Read the model definition and answer for the solid it produces. Units are mm, in the model's axes. A direction names the side the tool comes from. Coordinates: 2 decimals unless noted, no trailing zeros. Write each loop counter-clockwise with the first axis right and the second up, starting at its lowest first coordinate (ties: lowest second). Pieces come first, ordered by that corner, then holes. Notation, with made-up numbers: (72.25, -7.5) -> (115.25, -7.5) arc R24 cw to (115.25, 26.5) -> close; hole circle Ø6 at (30.25, -13). An arc over 180 degrees is marked (long way). Write item = value, one per line. Start each with the question number.
1) Section A-A (y = 11.43) is taken. Count the separate pieces of the cut face and the enclosed holes in it, plus the area to 3 significant figures.
2) Section B-B (y = 45.72) is taken. Determine the outline of the cut face in (x, z).
3) For a pull along X with two mould halves and no side action, classify faces 1 (the face through (143.192, 23.568, -63.64)), 2 (the face through (117.675, 46.483, -108.179)), 3 (the face through (23.976, 23.568, 4.834)), 4 (the face through (102, 50.8, -108)) as released by +X, released by -X, zero draft, split by the parting line, or undercut.
4) A tool of negligible diameter and unlimited length cuts with its end or side. For faces 5 (the face through (120.968, 3, -76)), 6 (the face through (145.15, 23.57, -76.71)), 7 (the face through (146.24, 20.51, -65.41)), 8 (the face through (34.3, 23.6, 13.1)), 9 (the face through (102, 28, -114.617)), from which of +Z, -Z, +X, -X, +Y, -Y can it reach the whole face along a straight path? Write none if from no direction.
5) Flat-ended cylindrical pins translate along their axes: pin 1 Ø10 at (y, z) = (24.5, -109) entering from +X; pin 2 Ø20 at (x, z) = (21, 7) entering from +Y (3 decimals); pin 3 Ø7 at (x, y) = (109, 2.5) entering from -Z; pin 4 Ø4.5 at (x, y) = (88.58, 11.43) entering from -Z. Find the tip coordinate at first contact, or state that the pin passes through.
6) Find the intervals of material crossed by line 1 along Y through (x, z) = (-4, -113.5); line 2 along Z through (x, y) = (147.25, 19.05); line 3 along Z through (x, y) = (83, 9), in increasing order. Write a range as from..to.
7) Section C-C (x = 110) is taken. Determine the outline of the cut face in (y, z), plus the area to 3 significant figures.
8) Section D-D (z = -98) is taken. Determine the outline of the cut face in (x, y), plus the area to 3 significant figures.
from build123d import *

# Parameters (mm, degrees)
SKETCH1_W           = 127.635
SKETCH1_H           = 127.635
MAIN_PLATE_DEPTH    = 6.35
SKETCH9_R           = 85.725
BOSS_EXTRUDE1_DEPTH = 6.35
SKETCH10_R          = 95.25
SKETCH10_R_2        = 85.4075
CUT_EXTRUDE1_DEPTH  = 167.64
SKETCH18_R          = 85.4075
SKETCH18_R_2        = 79.375
BOSS_EXTRUDE2_DEPTH = 38.1
SKETCH15_R          = 2.159
CUT_EXTRUDE3_DEPTH  = 88.9
CIRPATTERN1_COUNT   = 3
SKETCH23_R          = 79.375
CUT_EXTRUDE6_DEPTH  = 111.600000066
SKETCH24_W          = 38.1
SKETCH24_H          = 50.8
CUT_EXTRUDE7_DEPTH  = 7.35
SKETCH25_W          = 38.1
SKETCH25_H          = 12.7
BOSS_EXTRUDE3_DEPTH = 44.45
SKETCH26_R          = 2.54
CUT_EXTRUDE8_DEPTH  = 44.45


with BuildPart() as part:
    # Sketch1 → Main Plate (new body)
    with BuildSketch(Plane(origin=(0, 0, 0), x_dir=(1, 0, 0), z_dir=(0, 1, 0))):
        with Locations((63.8175, 63.8175)):
            Rectangle(SKETCH1_W, SKETCH1_H)
    extrude(amount=MAIN_PLATE_DEPTH)

    # Sketch9 → Boss-Extrude1 (add)
    with BuildSketch(Plane(origin=(0, 6.35, 0), x_dir=(1, 0, 0), z_dir=(0, 1, 0))):
        with Locations((63.8175, 63.8175)):
            Circle(SKETCH9_R)
    extrude(amount=-BOSS_EXTRUDE1_DEPTH)

    # Sketch10 → Cut-Extrude1 (cut)
    with BuildSketch(Plane(origin=(0, 6.35, 0), x_dir=(1, 0, 0), z_dir=(0, 1, 0))):
        with Locations((63.8175, 63.8175)):
            Circle(SKETCH10_R)
        with Locations((63.8175, 63.8175)):
            Circle(SKETCH10_R_2, mode=Mode.SUBTRACT)
    extrude(amount=-CUT_EXTRUDE1_DEPTH, mode=Mode.SUBTRACT)

    # Sketch18 → Boss-Extrude2 (add)
    with BuildSketch(Plane(origin=(0, 3.175, 0), x_dir=(1, 0, 0), z_dir=(0, 1, 0))):
        with Locations((63.8175, 63.8175)):
            Circle(SKETCH18_R)
        with Locations((63.8175, 63.8175)):
            Circle(SKETCH18_R_2, mode=Mode.SUBTRACT)
    extrude(amount=BOSS_EXTRUDE2_DEPTH)

    # Sketch15 → Cut-Extrude3 (cut)
    with BuildSketch(Plane(origin=(166.221610148, -6.35, 178.614251028), x_dir=(-0.866025404, 0, -0.5), z_dir=(0.5, 0, -0.866025404))):
        with Locations((209.900436354, 25.4)):
            Circle(SKETCH15_R)
        with Locations((209.900436354, 41.275)):
            Circle(SKETCH15_R)
    cut_extrude3 = extrude(amount=CUT_EXTRUDE3_DEPTH, mode=Mode.SUBTRACT)

    # CirPattern1: Cut-Extrude3 ×3 about axis
    cirpattern1_axis = Axis((63.8175, -161.29, -63.8175), (0, 1, 0))
    for i in range(1, CIRPATTERN1_COUNT):
        add(cut_extrude3.rotate(cirpattern1_axis, i * 360 / CIRPATTERN1_COUNT), mode=Mode.SUBTRACT)

    # Sketch23 → Cut-Extrude6 (cut)
    with BuildSketch(Plane(origin=(0, 6.35, 0), x_dir=(1, 0, 0), z_dir=(0, 1, 0))):
        with Locations((63.8175, 63.8175)):
            Circle(SKETCH23_R)
        with BuildLine():
            Line((13.678739997, 125.352005526), (7.552270878, 134.237860218))
            Line((7.552270878, 134.237860218), (-19.267108419, 125.320629884))
            Line((-19.267108419, 125.320629884), (-48.79695837, 60.397770071))
            Line((-48.79695837, 60.397770071), (-9.884344094, 7.052469015))
            Line((-9.884344094, 7.052469015), (6.959175986, -7.46308736))
            Line((6.959175986, -7.46308736), (13.678739997, 2.282994474))
            ThreePointArc((13.678739997, 2.282994474), (-15.5575, 63.8175), (13.678739997, 125.352005526))
        make_face()
        with BuildLine():
            Line((142.177324996, 76.471687114), (152.935935453, 77.334437661))
            Line((152.935935453, 77.334437661), (158.623077101, 105.019316613))
            Line((158.623077101, 105.019316613), (117.163156193, 163.054346747))
            Line((117.163156193, 163.054346747), (51.508463168, 156.027684783))
            Line((51.508463168, 156.027684783), (30.515862556, 148.698546693))
            Line((30.515862556, 148.698546693), (35.596435007, 138.00619264))
            ThreePointArc((35.596435007, 138.00619264), (103.505, 132.558266425), (142.177324996, 76.471687114))
        make_face()
        with BuildLine():
            Line((35.596435007, -10.37119264), (30.964293669, -20.119797879))
            Line((30.964293669, -20.119797879), (52.096531318, -38.887446496))
            Line((52.096531318, -38.887446496), (123.086302178, -31.999616818))
            Line((123.086302178, -31.999616818), (149.828380926, 28.372346201))
            Line((149.828380926, 28.372346201), (153.977461458, 50.217040667))
            Line((153.977461458, 50.217040667), (142.177324996, 51.163312886))
            ThreePointArc((142.177324996, 51.163312886), (103.505, -4.923266425), (35.596435007, -10.37119264))
        make_face()
    extrude(amount=CUT_EXTRUDE6_DEPTH, mode=Mode.SUBTRACT)

    # Sketch24 → Cut-Extrude7 (cut, through all)
    with BuildSketch(Plane(origin=(0, 6.35, 0), x_dir=(1, 0, 0), z_dir=(0, 1, 0))):
        with Locations((101.9175, 76.5175)):
            Rectangle(SKETCH24_W, SKETCH24_H)
    extrude(amount=-CUT_EXTRUDE7_DEPTH, mode=Mode.SUBTRACT)

    # Sketch25 → Boss-Extrude3 (add)
    with BuildSketch(Plane(origin=(0, 6.35, 0), x_dir=(1, 0, 0), z_dir=(0, 1, 0))):
        with Locations((101.9175, 108.2675)):
            Rectangle(SKETCH25_W, SKETCH25_H)
    extrude(amount=BOSS_EXTRUDE3_DEPTH)

    # Sketch26 → Cut-Extrude8 (cut)
    with BuildSketch(Plane.XY.offset(-101.9175)):
        with Locations((115.2525, 45.72)):
            Circle(SKETCH26_R)
        with Locations((88.5825, 11.43)):
            Circle(SKETCH26_R)
    extrude(amount=-CUT_EXTRUDE8_DEPTH, mode=Mode.SUBTRACT)


solid = part.part
Answer key:
q1.separate_pieces = 5
q1.enclosed_holes = 0
q1.area = 888 mm^2
q2.outline = (82.87, -114.62) -> (112.71, -114.62) -> (112.71, -101.92) -> (82.87, -101.92) -> close; (117.79, -114.62) -> (120.97, -114.62) -> (120.97, -101.92) -> (117.79, -101.92) -> close
q3.face_1 = released by -X
q3.face_2 = undercut
q3.face_3 = released by +X
q3.face_4 = zero draft
q4.face_5 = +Y, -Y
q4.face_6 = -Z, -X, +Y
q4.face_7 = +X, -X
q4.face_8 = +Z, +X, +Y
q4.face_9 = -Z, +X, -X, +Y
q5.pin_1 = 120.97
q5.pin_2 = 41.275
q5.pin_3 = -138.36
q5.pin_4 = through
q6.line_1 = 0..6.35
q6.line_2 = -76.88..-65.98, -61.66..-50.76
q6.line_3 = -114.62..-101.92
q7.outline = (0, -135.66) -> (6.35, -135.66) -> (6.35, -114.62) -> (50.8, -114.62) -> (50.8, -101.92) -> (0, -101.92) -> close; (0, -51.12) -> (6.35, -51.12) -> (6.35, 8.03) -> (0, 8.03) -> close
q7.area = 1,150 mm^2
q8.outline = (-14.45, 0) -> (82.87, 0) -> (82.87, 6.35) -> (-14.45, 6.35) -> close; (120.97, 0) -> (142.09, 0) -> (142.09, 6.35) -> (120.97, 6.35) -> close
q8.area = 752 mm^2
